Build history of the part. All positions in model axes, mm. Round coordinates to 2 decimals unless told otherwise and drop trailing zeros. Write each loop counter-clockwise with the first axis right and the second up, starting at its lowest first coordinate (ties: lowest second). Pieces come first, ordered by that corner, then holes.
1) Saw through at A-A (x = 4.5). Write the cut outline in (y, z), plus the area to 3 significant figures.
2) Wall check: probe 1 along Z at (x, y) = (0, 2.7); probe 2 along X at (y, z) = (2, 0); probe 3 along X at (y, z) = (4, 6.5). Give the ranges that are in metal, low to high.
3) Saw through at C-C (y = 1.55). Write the cut outline in (x, z).
4) Pull direction Z, two halves, no side cores. Call faces 1 (the cylindrical face through (-12.668, 2.958, 7.175)), 2 (the flat face through (0, 6, -3)), 3 (the cylindrical face through (-0.1, 2.96, 4.31)), 4 (the cylindrical face through (3.785, 2.958, -2.066)): +Z half, -Z half, draft (parallel to the pull), parting line (faces both ways), or undercut.
5) Flat gauge pins, fed straight in: pin 1 (2 mm diameter, centred on x = 2, y = 2.5, fed in from +Z); pin 2 (2 mm diameter, centred on x = 5.5, y = 4, fed in from -Z); pin 3 (1.5 mm diameter, centred on y = 4, z = -8.5, fed in from +X). Where does each tip first touch, or does it go through?
6) Saw through at D-D (z = -9.56). Write the cut outline in (x, y).
7) Saw through at B-B (z = 4.78). Write the cut outline in (x, y), plus the area to 3 significant figures.
from build123d import *

# Parameters (mm, degrees)
BOSS_EXTRUDE1_DEPTH = 6
SKETCH3_R           = 2.5
CUT_EXTRUDE1_DEPTH  = 8


with BuildPart() as part:
    # Sketch2 → Boss-Extrude1 (new body)
    with BuildSketch(Plane(origin=(0, 0, 0), x_dir=(1, 0, 0), z_dir=(0, 1, 0))):
        with BuildLine():
            ThreePointArc((10.127144448, -0.134021967), (3.73256949, 2.155), (4.947505796, 8.837375343))
            ThreePointArc((4.947505796, 8.837375343), (0, 14.56), (-4.947505796, 8.837375343))
            ThreePointArc((-4.947505796, 8.837375343), (-3.73256949, 2.155), (-10.127144448, -0.134021967))
            ThreePointArc((-10.127144448, -0.134021967), (-12.609329879, -7.28), (-5.179638652, -8.703353377))
            ThreePointArc((-5.179638652, -8.703353377), (0, -4.31), (5.179638652, -8.703353377))
            ThreePointArc((5.179638652, -8.703353377), (12.609329879, -7.28), (10.127144448, -0.134021967))
        make_face()
    extrude(amount=BOSS_EXTRUDE1_DEPTH)

    # Sketch3 → Cut-Extrude1 (cut)
    with BuildSketch(Plane(origin=(0, 6, 0), x_dir=(1, 0, 0), z_dir=(0, 1, 0))):
        Circle(SKETCH3_R)
    extrude(amount=-CUT_EXTRUDE1_DEPTH, mode=Mode.SUBTRACT)


solid = part.part
Evaluation:
1. outline: (0, -11.74) - (6, -11.74) - (6, -8.42) - (0, -8.42) - close; (0, -1.14) - (6, -1.14) - (6, 6.86) - (0, 6.86) - close
1. area: 67.8 mm2
2. probe 1: z = -14.56 to -2.5, 2.5 to 4.31
2. probe 2: x = -6.11 to -2.5, 2.5 to 6.11
2. probe 3: x = -12.97 to -4.27, 4.27 to 12.97
3. outline: (-10.13, 0.13) arc R5.25 cw to (-4.95, -8.84) arc R5 ccw (long way) to (4.95, -8.84) arc R5.25 cw to (10.13, 0.13) arc R5 ccw (long way) to (5.18, 8.7) arc R5.25 cw to (-5.18, 8.7) arc R5 ccw (long way) to start; hole circle Ø5 at (0, 0)
4. face 1: parting line
4. face 2: draft
4. face 3: +Z half
4. face 4: undercut
5. pin 1: stops at z = 5.25
5. pin 2: stops at z = -11.74
5. pin 3: stops at x = 4.99
6. outline: (-5, 0) - (5, 0) - (5, 6) - (-5, 6) - close
7. outline: (-13.28, 0) - (-2.17, 0) - (-2.17, 6) - (-13.28, 6) - close; (2.17, 0) - (13.28, 0) - (13.28, 6) - (2.17, 6) - close
7. area: 133 mm2
